Autodesk Inventor part; units mm, degrees
ref_plane "YZ Plane" through (0, 0, 0) normal (1, 0, 0) x (0, 1, 0)
ref_plane "XZ Plane" through (0, 0, 0) normal (0, 1, 0) x (-1, 0, 0)
ref_plane "XY Plane" through (0, 0, 0) normal (0, 0, 1) x (1, 0, 0)
sketch "Sketch1" plane through (0, 0, 0) normal (0, 1, 0) x (-1, 0, 0)
  line L0 (0, 0) -> (12.7, 0)
  line L1 (12.7, 0) -> (12.7, 13.716)
  line L2 (12.7, 13.716) -> (0, 13.716)
  line L3 (0, 13.716) -> (0, 0)
  dimension "d0" = 12.7
  dimension "d1" = 13.716
extrude "Extrusion1" add sketch "Sketch1" along normal blind 2.286
sketch "Sketch2" plane through (-12.7, 0, 13.716) normal (0, 0, 1) x (1, 0, 0)
  line L0 (0, 2.286) -> (12.7, 2.286)
  line L1 (0, 0) -> (0, 2.286)
  line L2 (0.762, 1.524) -> (1.524, 1.524)
  line L3 (1.524, 1.524) -> (1.524, 0.762)
  line L4 (1.524, 0.762) -> (0.762, 0.762)
  line L5 (0.762, 0.762) -> (0.762, 1.524)
  dimension "d4" = 0.762
  dimension "d5" = 0.762
  dimension "d6" = 0.762
  dimension "d7" = 0.762
extrude "Extrusion2" cut sketch "Sketch2" against normal blind 12.7
chamfer "Chamfer1" distance 0.254 angle 45 4 edges at (-11.938, 1.143, 13.716) (-11.557, 1.524, 13.716) (-11.176, 1.143, 13.716) (-11.557, 0.762, 13.716)
sketch "Sketch3" plane through (0, 0, 0) normal (0, 0, -1) x (-1, 0, 0)
  line L0 (11.938, 1.524) -> (11.176, 1.524)
  line L1 (11.938, 0.762) -> (11.938, 1.524)
  line L2 (11.176, 0.762) -> (11.938, 0.762)
  line L3 (11.176, 1.524) -> (11.176, 0.762)
  circle A0 centre (11.557, 1.143) radius 0.2335
  point P0 (11.557, 1.524)
  point P1 (11.176, 1.143)
extrude "Extrusion3" cut sketch "Sketch3" against normal blind 0.6477 contours A0
sketch "Sketch4" plane through (0, 0, 0) normal (0, -1, 0) x (1, 0, 0)
  line L0 (-12.7, 13.716) -> (0, 13.716)
  line L1 (-12.7, 0) -> (-12.7, 13.716)
  line L2 (-11.176, 13.462) -> (-11.176, 1.016)
  line L3 (-11.938, 13.462) -> (-11.938, 1.016)
  line L4 (-11.176, 1.016) -> (-11.938, 1.016)
  line L5 (-12.192, 9.906) -> (-10.922, 9.906)
  line L6 (-10.922, 9.906) -> (-10.922, 8.636)
  line L7 (-10.922, 8.636) -> (-12.192, 8.636)
  line L8 (-12.192, 8.636) -> (-12.192, 9.906)
  dimension "d18" = 0.508
  dimension "d19" = 1.27
  dimension "d20" = 1.27
  dimension "d21" = 3.81
extrude "Extrusion4" cut sketch "Sketch4" against normal blind 0.127 contours L5 L6 L7 L2 | L2 L7 L3 L5 | L3 L7 L8 L5
pattern_linear "Rectangular Pattern1" count 5 spacing 2.54 along (1, 0, 0) of "Extrusion2", "Chamfer1", "Extrusion3", "Extrusion4"
properties part number "Five Pin Plug"
Source: CAD feature listing. Evaluate the final solid. Frame: model axes, mm. A direction names the side the tool comes from. Give positions to 0.01 mm unless a question says otherwise; leave off trailing zeros. Order: outer loops, then holes, each group sorted by start corner. A loop starts at its lowest first (then second) coordinate and runs counter-clockwise, first axis right, second up. Notation, with made-up numbers: (4, 34) -> (55, 34) arc R29 ccw to (55, 61) -> close; hole circle Ø6 at (45, 59.25). An arc over 180 degrees is marked (long way). Write item = value, one per line.
Q1. Material intervals for line 1 (X direction, y = 1.2, z = 10.25); line 2 (Y direction, x = -11.25, z = 9.5); line 3 (Z direction, x = -11.5, y = 1.7), sorted ascending. Write a range as from..to.
Data:
line_1 = -12.7..-11.94, -11.18..-9.4, -8.64..-6.86, -6.1..-4.32, -3.56..-1.78, -1.02..0
line_2 = 0.13..0.76, 1.52..2.29
line_3 = 0..13.64
Q2. Set-up query: faces 5 (the face through (-12, 0.127, 9)), 6 (the face through (0, 1, 7)). Return all of +Z, -Z, +X, -X, +Y, -Y with unobstructed straight access to the full face (end or side cutting, diameter ignored); none if empty.
Data:
face_5 = -Y
face_6 = +Z, -Z, +X, +Y, -Y
Q3. Cut plane B-B, the plane x = -9. Output: boundary loops of the cut face in (y, z), and give its area (3 significant figures).
Data:
outline = (0, 0) -> (0.91, 0) -> (0.91, 0.65) -> (1.38, 0.65) -> (1.38, 0) -> (2.29, 0) -> (2.29, 13.72) -> (1.78, 13.72) -> (1.52, 13.46) -> (1.52, 1.02) -> (0.76, 1.02) -> (0.76, 13.46) -> (0.51, 13.72) -> (0, 13.72) -> (0, 9.91) -> (0.13, 9.91) -> (0.13, 8.64) -> (0, 8.64) -> close
area = 21.1 mm^2
Q4. Pull-direction query (Z, two-part tool) for faces 1 (the face through (-6, 0.127, 9)), 2 (the face through (-6, 1, 0)), 3 (the face through (-6, 2, 13.716)), 4 (the face through (-1, 0.127, 9)); classes: released by +Z, released by -Z, zero draft, split by the parting line, or undercut.
Data:
face_1 = undercut
face_2 = released by -Z
face_3 = released by +Z
face_4 = undercut
Q5. Cut plane A-A, the plane z = 6.75. Output: boundary loops of the cut face in (x, y).
Data:
outline = (-12.7, 0) -> (0, 0) -> (0, 2.29) -> (-12.7, 2.29) -> close; hole (-11.94, 0.76) -> (-11.18, 0.76) -> (-11.18, 1.52) -> (-11.94, 1.52) -> close; hole (-9.4, 0.76) -> (-8.64, 0.76) -> (-8.64, 1.52) -> (-9.4, 1.52) -> close; hole (-6.86, 0.76) -> (-6.1, 0.76) -> (-6.1, 1.52) -> (-6.86, 1.52) -> close; hole (-4.32, 0.76) -> (-3.56, 0.76) -> (-3.56, 1.52) -> (-4.32, 1.52) -> close; hole (-1.78, 0.76) -> (-1.02, 0.76) -> (-1.02, 1.52) -> (-1.78, 1.52) -> close
